Geometry: final body of the model. Coordinates: model frame, mm. A direction names the side the tool comes from. Round coordinates to 2 decimals unless told otherwise and drop trailing zeros. Write each loop counter-clockwise with the first axis right and the second up, starting at its lowest first coordinate (ties: lowest second). Pieces come first, ordered by that corner, then holes. Notation, with made-up numbers: (14, 89.25) -> (49, 89.25) arc R7 ccw to (49, 94.25) -> close; hole circle Ø3 at (-36.5, -26.75). An arc over 180 degrees is marked (long way). Use one line per item in the form item = value. Start each with the question number.
1. Reachability of faces 4 (the face through (82, 92, 0)), 5 (the face through (86.156, 91.491, 11.674)), 6 (the face through (84.547, 87.214, 5.127)) from +Z, -Z, +X, -X, +Y, -Y: full face, straight path, thin tool, end or side. Return the list, or none.
2. Pin query (flat end, axial travel): pin 1 Ø3 at (x, y) = (76.01, 95.13) entering from +Z; pin 2 Ø2 at (y, z) = (84.5, 2) entering from -X; pin 3 Ø8 at (y, z) = (98, 11) entering from -X; pin 4 Ø1 at (x, y) = (82, 95.5) entering from -Z. Return the tip coordinate at first contact, or that it passes through.
3. Draft query along X for faces 1 (the face through (76, 95, 9.9)), 2 (the face through (76.82, 76.88, 11.43)), 3 (the face through (79, 86, 13.4)). Return one class per face: pulls with the +X half, pulls with the -X half, needs draft (parallel to the pull), parting line crosses it, or undercut.
4. Line query: L1, parallel to X at y = 91.25, z = 5.75; L2, parallel to X at y = 91, z = 2.75; L3, parallel to Y at x = 85.5, z = 6.25. Output: solid intervals per line, ascending.
5. Cut plane A-A, the plane z = 4.5. Return the cut outline in (x, y).
Autodesk Inventor part; units mm, degrees
ref_plane "YZ Plane" through (0, 0, 0) normal (1, 0, 0) x (0, 1, 0)
ref_plane "XZ Plane" through (0, 0, 0) normal (0, 1, 0) x (-1, 0, 0)
ref_plane "XY Plane" through (0, 0, 0) normal (0, 0, 1) x (1, 0, 0)
sketch "스케치1" plane through (0, 0, 0) normal (0, 0, 1) x (1, 0, 0)
  circle A0 centre (77.7382, 82.3139) radius 1.75
  circle A1 centre (72.7611, 90.8713) radius 1.75
  circle A2 centre (86.2956, 87.2909) radius 1.75
  circle A3 centre (81.3185, 95.8484) radius 1.75
  circle A4 centre (79.5283, 89.0811) radius 11.15
  circle A5 centre (79.5283, 89.0811) radius 10.85
  circle A6 centre (79.5283, 89.0811) radius 1.6
  circle A7 centre (79.5283, 89.0811) radius 2.8
  circle A8 centre (79.5283, 89.0811) radius 2.5
  point P0 (0, 0)
  dimension "d0" = 0.3
  dimension "d3" = 3.2
extrude "돌출1" add sketch "스케치1" along normal blind 13.4 contours A5 | A7 | A8
sketch "스케치2" plane through (79.5283, 89.0811, 13.4) normal (0, 0, 1) x (1, 0, 0)
  circle A0 centre (0, 0) radius 10.85
  circle A1 centre (0, 0) radius 12.5
  dimension "d4" = 25
extrude "돌출2" add sketch "스케치2" against normal blind 4
chamfer "모따기1" distance 0.2 angle 45 1 edges at (68.6783, 89.0811, 0)
sketch "스케치3" plane through (79.5283, 89.0811, 0) normal (0, 0, -1) x (-1, 0, 0)
  circle A0 centre (0, 0) radius 1.6
  circle A1 centre (0, 0) radius 10.65
  circle A2 centre (0, 0) radius 3.2
  dimension "d13" = 6.4
extrude "돌출3" cut sketch "스케치3" against normal blind 12.5 contours A2
sketch "스케치5" plane through (79.5283, 89.0811, 13.4) normal (0, 0, 1) x (1, 0, 0)
  circle A0 centre (0, 0) radius 12.5
  circle A1 centre (-1.7902, -6.7672) radius 1.75
  circle A2 centre (-1.7902, -6.7672) radius 1.25
  circle A3 centre (3.5193, -6.051) radius 1.25
  circle A4 centre (6.7672, -1.7902) radius 1.25
  circle A5 centre (6.051, 3.5193) radius 1.25
  circle A6 centre (1.7902, 6.7672) radius 1.25
  circle A7 centre (-3.5193, 6.051) radius 1.25
  circle A8 centre (-6.7672, 1.7902) radius 1.25
  circle A9 centre (-6.051, -3.5193) radius 1.25
  dimension "d18" = 2.5
  dimension "d21" = 360
extrude "돌출5" cut sketch "스케치5" against normal blind 3.5 contours A3 | A5 | A7 | A9
sketch "스케치4" plane through (79.5283, 89.0811, 13.4) normal (0, 0, 1) x (1, 0, 0)
  circle A0 centre (1.7902, 6.7672) radius 1.75
  circle A1 centre (6.7672, -1.7902) radius 1.75
  circle A2 centre (-6.7672, 1.7902) radius 1.75
  circle A3 centre (-1.7902, -6.7672) radius 1.75
extrude "돌출4" add sketch "스케치4" against normal blind 3
properties part number "gear_support" material "고무, 검은색"
Outcome:
q1.face_4 = -Z, +X, -X, +Y, -Y
q1.face_5 = +Z
q1.face_6 = -Z
q2.pin_1 = 13.4
q2.pin_2 = 69.29
q2.pin_3 = 68.04
q2.pin_4 = 10.4
q3.face_1 = undercut
q3.face_2 = parting line crosses it
q3.face_3 = needs draft
q4.L1 = 68.9 to 71.05, 74.47 to 77.18, 81.88 to 90.16
q4.L2 = 68.85 to 71.02, 74.51 to 76.97, 82.09 to 90.21
q4.L3 = 80.02 to 85.73, 88.85 to 98.14
q5.outline = circle Ø21.7 at (79.53, 89.08); hole circle Ø3.5 at (72.76, 90.87); hole circle Ø3.5 at (77.74, 82.31); hole circle Ø6.4 at (79.53, 89.08); hole circle Ø3.5 at (81.32, 95.85); hole circle Ø3.5 at (86.3, 87.29)
